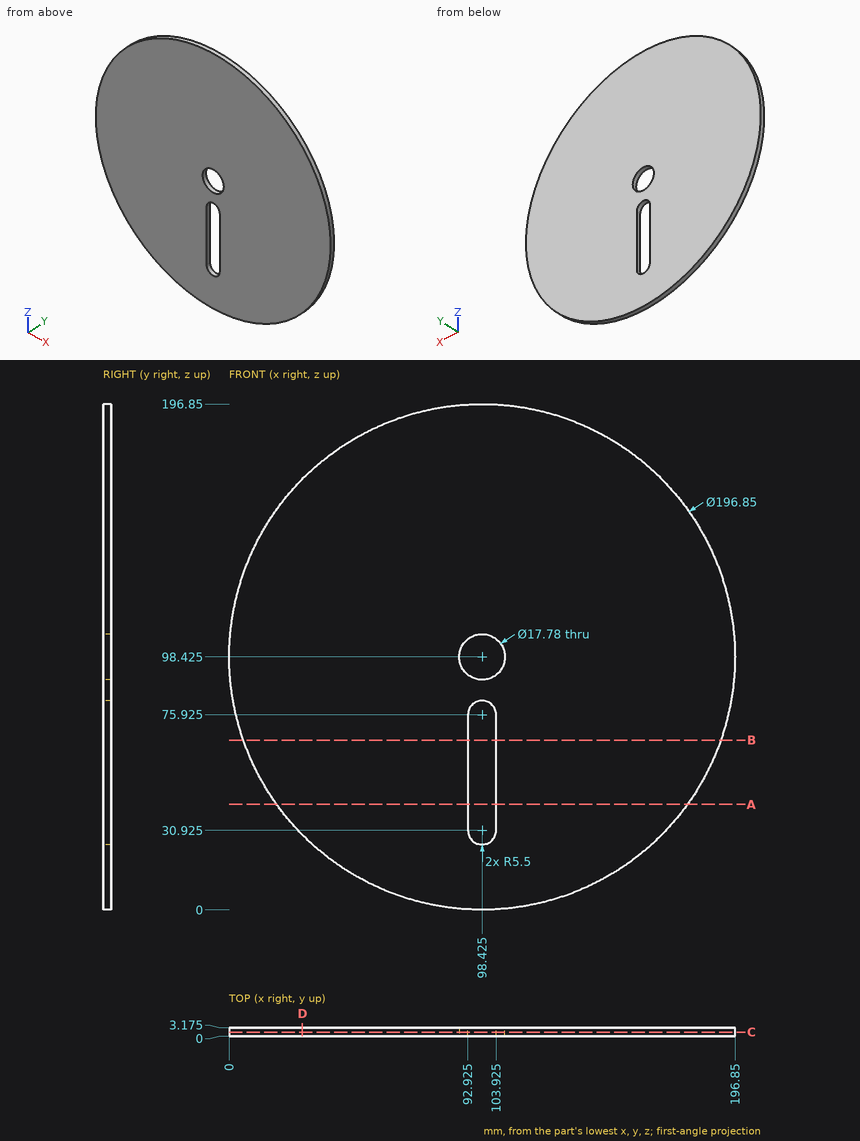
Source: three-view drawing plus pictorial views. Frame: mm from the lowest corner of the part. Give positions to 0.01 mm unless a question says otherwise; leave off trailing zeros. Order: outer loops, then holes, each group sorted by start corner. A loop starts at its lowest first (then second) coordinate and runs counter-clockwise, first axis right, second up. Notation, with made-up numbers: (12, 89) - (71, 89) arc R22 ccw to (71, 121) - close; hole circle Ø8 at (78.5, 89). An arc over 180 degrees is marked (long way). Put each result on its own line as item: value.
Item 1: Section query B-B, the plane z = 66. Return loops of the section in (x, y) (3 decimals), then the cut area to 3 significant figures.
Found:
outline: (5.494, 0) - (92.925, 0) - (92.925, 3.175) - (5.494, 3.175) - close; (103.925, 0) - (191.356, 0) - (191.356, 3.175) - (103.925, 3.175) - close
area: 555 mm^2
Item 2: Ray query, L1, parallel to X at y = 3.05, z = 99; L2, parallel to X at y = 1.5, z = 170; L3, parallel to X at y = 0.7, z = 25. Return the intervals inside material, ascending. Write a range as from..to.
Found:
L1: x = 0..89.55, 107.3..196.85
L2: x = 30.86..165.99
L3: x = 32.88..163.97
Item 3: Section query C-C, the plane y = 1.55. Return loops of the section in (x, z) (3 decimals).
Found:
outline: circle Ø196.85 at (98.425, 98.425); hole circle Ø17.78 at (98.425, 98.425); hole (92.925, 30.925) arc R5.5 ccw to (103.925, 30.925) - (103.925, 75.925) arc R5.5 ccw to (92.925, 75.925) - close
Item 4: Section query D-D, the plane x = 28.5. Return loops of the section in (y, z) (3 decimals).
Found:
outline: (0, 29.158) - (3.175, 29.158) - (3.175, 167.692) - (0, 167.692) - close
Item 5: Section query A-A, the plane z = 41. Return loops of the section in (x, y) (3 decimals).
Found:
outline: (18.488, 0) - (92.925, 0) - (92.925, 3.175) - (18.488, 3.175) - close; (103.925, 0) - (178.362, 0) - (178.362, 3.175) - (103.925, 3.175) - close
Item 6: Contact query for a flat-ended pin moving along its axis: pin 1 (20.5 mm diameter, centred on x = 98.425, z = 98.425, fed in from -Y). Output: stop coordinate, or through.
Found:
pin 1: stops at y = 0
